```python
from build123d import *

# Parameters (mm, degrees)
F0_W     = 57.15
F0_H     = 57.15
F1_DEPTH = 88.9
F2_W     = 23.8125
F2_H     = 23.8125
F3_DEPTH = 76.2
F4_W     = 23.8125
F4_H     = 23.8125
F5_DEPTH = 76.2
F6_W     = 24.340702
F6_H     = 21.549652
F7_DEPTH = 76.2
F8_W     = 22.018882
F8_H     = 21.008313
F9_DEPTH = 76.2


with BuildPart() as f1:
    # F0 (on Top) → F1 (new body)
    with BuildSketch(Plane.XY):
        Rectangle(F0_W, F0_H)
    extrude(amount=F1_DEPTH)

    # F2 (on face) → F3 (cut)
    with BuildSketch(Plane.XY.offset(88.9)):
        with Locations((13.726034, 13.655303)):
            Rectangle(F2_W, F2_H)
    extrude(amount=-F3_DEPTH, mode=Mode.SUBTRACT)

    # F4 (on face) → F5 (cut)
    with BuildSketch(Plane.XY.offset(88.9)):
        with Locations((-11.932438, 13.372463)):
            Rectangle(F4_W, F4_H)
    extrude(amount=-F5_DEPTH, mode=Mode.SUBTRACT)

    # F6 (on face) → F7 (cut)
    with BuildSketch(Plane.XY.offset(88.9)):
        with Locations((-12.170351, -15.019511)):
            Rectangle(F6_W, F6_H)
    extrude(amount=-F7_DEPTH, mode=Mode.SUBTRACT)

    # F8 (on face) → F9 (cut)
    with BuildSketch(Plane.XY.offset(88.9)):
        with Locations((14.791763, -14.032443)):
            Rectangle(F8_W, F8_H)
    extrude(amount=-F9_DEPTH, mode=Mode.SUBTRACT)


solid = f1.part
```
Geometry check sheet. Reference: the model listing, model coordinates, mm. A direction names the side the tool comes from. Round coordinates to 2 decimals unless told otherwise and drop trailing zeros. Loops run counter-clockwise (first coordinate to the right, second up) from the corner with the lowest first, then second, coordinate; pieces in that order, holes last. Notation, with made-up numbers: (-39, 87) - (-19, 87) arc R15 cw to (-19, 96) - close; hole circle Ø4 at (-1.5, 38.25). An arc over 180 degrees is marked (long way). Write item = value, one per line. Start each with the question number.
1. Thickness scan on line 1 (X direction, y = 5.5, z = 17.5) (3 decimals); line 2 (Y direction, x = -12, z = 41.5) (3 decimals); line 3 (Y direction, x = 11, z = 52.5) (3 decimals). Record the ranges inside material, lowest first.
2. Set-up check for faces 4 (the face through (25.632, 13, 51)), 5 (the face through (-28.575, 0, 44)): record each of +Z, -Z, +X, -X, +Y, -Y from which the full face is reachable in a straight line by a thin tool's end or side.
3. Section check C-C on y = -19. Enter the section's corners in (x, z) (3 decimals), then the cut area to 3 significant figures.
4. Depth check by flat-ended pin: pin 1 (12 mm diameter, centred on x = -11.5, y = 8, fed in from +Z). Enter the tip coordinate at first touch or a pass-through.
5. Section check B-B on x = 17. Enter the section's corners in (y, z) (3 decimals).
6. Section check A-A on z = 46. Enter the section's corners in (x, y) (3 decimals).
7. Mould release check, pull along Y, two halves, no side actions. Record for faces 1 (the face through (0, 28.575, 44)), 2 (the face through (-12, -25.794, 51)), 3 (the face through (-4, -4, 88.9)): released by +Y, released by -Y, zero draft, split by the parting line, or undercut.
Working result:
q1.line_1 = -28.575 to -23.839, -0.026 to 1.82, 25.632 to 28.575
q1.line_2 = -28.575 to -25.794, -4.245 to 1.466, 25.279 to 28.575
q1.line_3 = -28.575 to -24.537, -3.528 to 1.749, 25.562 to 28.575
q2.face_4 = +Z
q2.face_5 = +Z, -Z, -X, +Y, -Y
q3.outline = (-28.575, 0) - (28.575, 0) - (28.575, 88.9) - (25.801, 88.9) - (25.801, 12.7) - (3.782, 12.7) - (3.782, 88.9) - (0, 88.9) - (0, 12.7) - (-24.341, 12.7) - (-24.341, 88.9) - (-28.575, 88.9) - close
q3.area = 1,550 mm^2
q4.pin_1 = 12.7
q5.outline = (-28.575, 0) - (28.575, 0) - (28.575, 88.9) - (25.562, 88.9) - (25.562, 12.7) - (1.749, 12.7) - (1.749, 88.9) - (-3.528, 88.9) - (-3.528, 12.7) - (-24.537, 12.7) - (-24.537, 88.9) - (-28.575, 88.9) - close
q6.outline = (-28.575, -28.575) - (28.575, -28.575) - (28.575, 28.575) - (-28.575, 28.575) - close; hole (-24.341, -25.794) - (0, -25.794) - (0, -4.245) - (-24.341, -4.245) - close; hole (-23.839, 1.466) - (-0.026, 1.466) - (-0.026, 25.279) - (-23.839, 25.279) - close; hole (1.82, 1.749) - (25.632, 1.749) - (25.632, 25.562) - (1.82, 25.562) - close; hole (3.782, -24.537) - (25.801, -24.537) - (25.801, -3.528) - (3.782, -3.528) - close
q7.face_1 = released by +Y
q7.face_2 = undercut
q7.face_3 = zero draft
